from build123d import *

# Parameters (mm, degrees)
F0_W     = 40
F0_H     = 30
F0_R     = 2.5
F1_DEPTH = 5
F3_DEPTH = 31
F4_R     = 5


with BuildPart() as f1:
    # F0 (on Front) → F1 (new body)
    with BuildSketch(Plane.XZ):
        Rectangle(F0_W, F0_H)
        with Locations((-11, 0)):
            Circle(F0_R, mode=Mode.SUBTRACT)
        with Locations((11, 0)):
            Circle(F0_R, mode=Mode.SUBTRACT)
    extrude(amount=F1_DEPTH)

    # F2 (on face) → F3 (cut)
    with BuildSketch(Plane(origin=(0, 0, -15), x_dir=(1, 0, 0), z_dir=(0, 0, -1))):
        with BuildLine():
            Line((-1.5, 0), (1.5, 0))
            ThreePointArc((1.5, 0), (0, 1.5), (-1.5, 0))
        make_face()
    extrude(amount=-F3_DEPTH, mode=Mode.SUBTRACT)

    # F4
    f4_edges = [f1.edges().sort_by_distance(p)[0] for p in [
        (20, -2.5, -15),
        (-20, -2.5, -15),
        (20, -2.5, 15),
        (-20, -2.5, 15),
    ]]
    fillet(f4_edges, radius=F4_R)


solid = f1.part
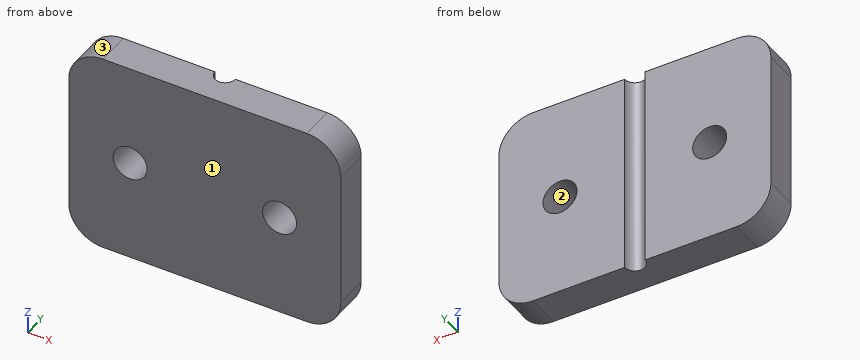
Work out the finished part from the listing and answer in its coordinate system (mm). Face numbers are marked on the shaded views. Round coordinates to 2 decimals unless told otherwise and drop trailing zeros. Loops run counter-clockwise (first coordinate to the right, second up) from the corner with the lowest first, then second, coordinate; pieces in that order, holes last. Notation, with made-up numbers: M 38,76.25 L 88,76.25 A20 cw 88,90.25 Z; hole C -23,-7 d3. An arc over 180 degrees is marked long. One line per question, with ' | ' between items. Start each with the question number.
(1) For a pull along X with two mould halves and no side action, classify the marked faces 1, 2 and 3 as released by +X, released by -X, zero draft, split by the parting line, or undercut.
(2) A cutting plane is placed at C-C on y = -0.75. Write down the section's boundary in (x, z).
(3) A cutting plane is placed at B-B on x = 13. Write down the section's boundary in (y, z).
(4) Find the intervals of material crossed by line 1 (Z direction, x = 11, y = -2.7); line 2 (X direction, y = -0.65, z = -5.5); line 3 (Z direction, x = 10, y = -0.8), in increasing order.
(5) A cutting plane is placed at D-D on y = -4.35. Write down the section's boundary in (x, z), plus the area to 3 significant figures.
(6) A cutting plane is placed at A-A on z = 0. Write down the section's boundary in (x, y).
Geometry check:
1) face 1: zero draft | face 2: undercut | face 3: released by -X
2) outline: M -20,-10 A5 ccw -15,-15 L -1.3,-15 L -1.3,15 L -15,15 A5 ccw -20,10 Z; M 1.3,-15 L 15,-15 A5 ccw 20,-10 L 20,10 A5 ccw 15,15 L 1.3,15 Z; hole C -11,0 d5; hole C 11,0 d5
3) outline: M -5,-15 L 0,-15 L 0,-1.5 L -5,-1.5 Z; M -5,1.5 L 0,1.5 L 0,15 L -5,15 Z
4) line 1: z = -15 to -2.5, 2.5 to 15 | line 2: x = -20 to -1.35, 1.35 to 20 | line 3: z = -15 to -2.29, 2.29 to 15
5) outline: M -20,-10 A5 ccw -15,-15 L 15,-15 A5 ccw 20,-10 L 20,10 A5 ccw 15,15 L -15,15 A5 ccw -20,10 Z; hole C -11,0 d5; hole C 11,0 d5 | area: 1,140 mm²
6) outline: M -20,-5 L -13.5,-5 L -13.5,0 L -20,0 Z; M -8.5,-5 L 8.5,-5 L 8.5,0 L 1.5,0 A1.5 cw -1.5,0 L -8.5,0 Z; M 13.5,-5 L 20,-5 L 20,0 L 13.5,0 Z
